For this review, use the dimensioned drawing (mm, ordinates from the lowest corner) and the shaded views. A direction names the side the tool comes from. Give positions to 0.01 mm unless a question says otherwise; leave off trailing zeros. Loops run counter-clockwise (first coordinate to the right, second up) from the corner with the lowest first, then second, coordinate; pieces in that order, holes last. Notation, with made-up numbers: (-0.5, 69.25) -> (5.5, 69.25) arc R10 ccw to (5.5, 80.25) -> close; hole circle Ø3 at (40.5, 87). An arc over 180 degrees is marked (long way). Write each question's results on one line, items separated by ' | '. Start each with the question number.
Q1. Wall thickness on L1, parallel to Z at x = 56.5, y = 60.5 (3 decimals); L2, parallel to Z at x = 56, y = 21; L3, parallel to Y at x = 60.5, z = 5: over which ranges is each line inside the solid? List them lowest first. Write a range as [from, to].
Q2. We need section B-B (x = 56). Write out the cut boundary in (y, z).
Q3. Mouldability with a two-part tool opening along X and no side actions: class the marked faces 5, 6 and 7 as released by +X, released by -X, zero draft, split by the parting line, or undercut.
Q4. We need section D-D (x = 21.5). Write out the cut boundary in (y, z), plus the area to 3 significant figures.
Q5. We need section C-C (z = 31). Write out the cut boundary in (x, y).
Q6. We need section A-A (y = 13.5). Write out the cut boundary in (x, z).
Q7. Machinability: for the marked faces 1, 2, 3 and 4, which of the approach directions +Z, -Z, +X, -X, +Y, -Y give a long, thin tool a straight path to every point of the face, cutting with its end or side? Answer none if there is none.
Q8. Insertion check: pin 1 Ø5 at (x, z) = (49.5, 5) entering from -Y; pin 2 Ø3 at (x, y) = (20, 26) entering from -Z; pin 3 Ø4.5 at (x, y) = (18.5, 49.5) entering from +Z. Each pin has a flat end and moves straight along its axis. Give the tip position at first contact, or say it passes through.
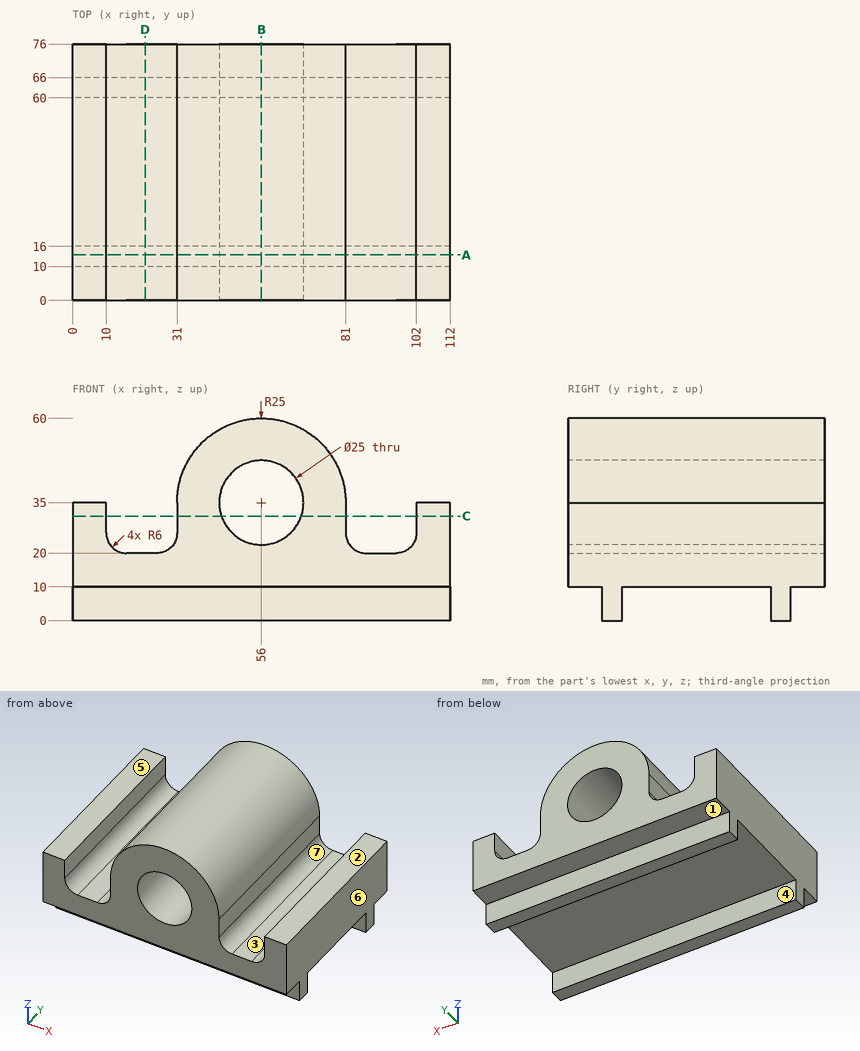
Output:
1) L1: [0, 22.51], [47.49, 59.995] | L2: [10, 22.5], [47.5, 60] | L3: [10, 16], [60, 66]
2) outline: (0, 10) -> (10, 10) -> (10, 0) -> (16, 0) -> (16, 10) -> (60, 10) -> (60, 0) -> (66, 0) -> (66, 10) -> (76, 10) -> (76, 22.5) -> (0, 22.5) -> close; (0, 47.5) -> (76, 47.5) -> (76, 60) -> (0, 60) -> close
3) face 5: zero draft | face 6: released by +X | face 7: undercut
4) outline: (0, 10) -> (10, 10) -> (10, 0) -> (16, 0) -> (16, 10) -> (60, 10) -> (60, 0) -> (66, 0) -> (66, 10) -> (76, 10) -> (76, 20) -> (0, 20) -> close | area: 880 mm2
5) outline: (0, 0) -> (10, 0) -> (10, 76) -> (0, 76) -> close; (31, 0) -> (44.16, 0) -> (44.16, 76) -> (31, 76) -> close; (67.84, 0) -> (81, 0) -> (81, 76) -> (67.84, 76) -> close; (102, 0) -> (112, 0) -> (112, 76) -> (102, 76) -> close
6) outline: (0, 0) -> (112, 0) -> (112, 35) -> (102, 35) -> (102, 26) arc R6 cw to (96, 20) -> (87, 20) arc R6 cw to (81, 26) -> (81, 35) arc R25 ccw to (31, 35) -> (31, 26) arc R6 cw to (25, 20) -> (16, 20) arc R6 cw to (10, 26) -> (10, 35) -> (0, 35) -> close; hole circle Ø25 at (56, 35)
7) face 1: -Z, +X, -X, +Y | face 2: +Z, +X, +Y, -Y | face 3: +Z, +Y, -Y | face 4: -Z, +X, -X
8) pin 1: y = 10 | pin 2: z = 10 | pin 3: z = 20
